For this review, take the finished solid that the model builds, in its own axes (mm). A direction names the side the tool comes from. Coordinates: 2 decimals unless noted, no trailing zeros. Order: outer loops, then holes, each group sorted by start corner. A loop starts at its lowest first (then second) coordinate and runs counter-clockwise, first axis right, second up. Notation, with made-up numbers: (81.25, 21) -> (140.25, 21) arc R33 ccw to (140.25, 60) -> close; hole circle Ø5 at (82, 22.5). An arc over 180 degrees is marked (long way). Write item = value, one per line. Start each with the question number.
1) Consider section A-A on y = 0. Give the boundary of the cut face in (x, z), and give its area (3 significant figures).
2) Machinability: for faces 1 (the face through (-4, 5, 2)), 2 (the face through (7, -4, 10)), 3 (the face through (4.93, -3.91, 7.46)), which of the approach directions +Z, -Z, +X, -X, +Y, -Y give a long, thin tool a straight path to every point of the face, cutting with its end or side? Answer none if there is none.
3) Insertion check: pin 1 Ø10 at (x, y) = (7.5, 6.5) entering from +Z; pin 2 Ø1.5 at (x, z) = (-5.5, 9) entering from +Y; pin 3 Ø5.5 at (y, z) = (3.5, 2.5) entering from -X; pin 4 Ø2.5 at (x, y) = (0, 0) entering from +Z. Each pin has a flat end and moves straight along its axis. Give the tip position at first contact, or say it passes through.
4) Wall thickness on probe 1 along Y at (x, z) = (0.25, 3.25); probe 2 along X at (y, z) = (9, 2.25); probe 3 along X at (y, z) = (3.75, 1.5): over which ranges is each line inside the solid? List them lowest first. Write a range as [from, to].
5) Consider section B-B on x = -9.25. Give the boundary of the cut face in (y, z), and give its area (3 significant figures).
6) Consider section C-C on x = 5.75. Give the boundary of the cut face in (y, z), and give its area (3 significant figures).
7) Draft analysis for pull direction X (two halves, no side actions). For faces 4 (the face through (0, 8, 10)), 5 (the face through (-11.99, 0.53, 2.54)), 6 (the face through (2.5, 0.2, 5)), state which applies: +X half, -X half, draft (parallel to the pull), parting line (faces both ways), or undercut.
8) Consider section D-D on z = 5.75. Give the boundary of the cut face in (x, y), and give its area (3 significant figures).
from build123d import *

# Parameters (mm, degrees)
BOSS_EXTRUDE1_DEPTH     = 5
SKETCH3_R               = 2
BOSS_EXTRUDE2_DEPTH     = 5
SKETCH4_R               = 2
CUT_EXTRUDE1_DEPTH      = 6
CUT_EXTRUDE1_DEPTH_BACK = 6
SKETCH5_R               = 12
SKETCH5_R_2             = 10
BOSS_EXTRUDE3_DEPTH     = 5


with BuildPart() as part:
    # Sketch1 → Boss-Extrude1 (new body)
    with BuildSketch(Plane.XY):
        with BuildLine():
            Line((4, 2.309401077), (4, 8))
            ThreePointArc((4, 8), (0, 12), (-4, 8))
            Line((-4, 8), (-4, 2.309401077))
            Line((-4, 2.309401077), (-8.92820323, -0.535898385))
            ThreePointArc((-8.92820323, -0.535898385), (-10.392304845, -6), (-4.92820323, -7.464101615))
            Line((-4.92820323, -7.464101615), (0, -4.618802154))
            Line((0, -4.618802154), (4.92820323, -7.464101615))
            ThreePointArc((4.92820323, -7.464101615), (10.392304845, -6), (8.92820323, -0.535898385))
            Line((8.92820323, -0.535898385), (4, 2.309401077))
        make_face()
    extrude(amount=BOSS_EXTRUDE1_DEPTH)

    # Sketch3 → Boss-Extrude2 (add)
    with BuildSketch(Plane.XY.offset(5)):
        with Locations((0, 8)):
            Circle(SKETCH3_R)
        with Locations((6.92820323, -4)):
            Circle(SKETCH3_R)
        with Locations((-6.92820323, -4)):
            Circle(SKETCH3_R)
        Circle(SKETCH3_R)
    extrude(amount=BOSS_EXTRUDE2_DEPTH)

    # Sketch4 → Cut-Extrude1 (cut, two sides)
    with BuildSketch(Plane.XY.offset(5)) as cut_extrude1_sk:
        Circle(SKETCH4_R)
    extrude(amount=CUT_EXTRUDE1_DEPTH, mode=Mode.SUBTRACT)
    extrude(cut_extrude1_sk.sketch, amount=-CUT_EXTRUDE1_DEPTH_BACK, mode=Mode.SUBTRACT)

    # Sketch5 → Boss-Extrude3 (add)
    with BuildSketch(Plane.XY.offset(5)):
        Circle(SKETCH5_R)
        Circle(SKETCH5_R_2, mode=Mode.SUBTRACT)
    extrude(amount=-BOSS_EXTRUDE3_DEPTH)


solid = part.part
Answer sheet:
q1.outline = (-12, 0) -> (-10, 0) -> (-10, 5) -> (-12, 5) -> close; (-8, 0) -> (-2, 0) -> (-2, 5) -> (-8, 5) -> close; (2, 0) -> (8, 0) -> (8, 5) -> (2, 5) -> close; (10, 0) -> (12, 0) -> (12, 5) -> (10, 5) -> close
q1.area = 80.0 mm2
q2.face_1 = +Z, -Z
q2.face_2 = +Z, +X, -X, +Y, -Y
q2.face_3 = +Z
q3.pin_1 = 5
q3.pin_2 = -2.12
q3.pin_3 = -11.98
q3.pin_4 = through
q4.probe_1 = [-12, -10], [-4.76, -1.98], [1.98, 12]
q4.probe_2 = [-7.94, -4.36], [-3.87, 3.87], [4.36, 7.94]
q4.probe_3 = [-11.4, -9.27], [-4, 4], [9.27, 11.4]
q5.outline = (-7.64, 0) -> (-0.74, 0) -> (-0.74, 5) -> (-7.64, 5) -> close; (3.8, 0) -> (7.64, 0) -> (7.64, 5) -> (3.8, 5) -> close
q5.area = 53.7 mm2
q6.outline = (-10.53, 0) -> (-8.18, 0) -> (-8.18, 5) -> (-10.53, 5) -> close; (-7.82, 0) -> (1.3, 0) -> (1.3, 5) -> (-2.38, 5) -> (-2.38, 10) -> (-5.62, 10) -> (-5.62, 5) -> (-7.82, 5) -> close; (8.18, 0) -> (10.53, 0) -> (10.53, 5) -> (8.18, 5) -> close
q6.area = 85.3 mm2
q7.face_4 = draft
q7.face_5 = parting line
q7.face_6 = undercut
q8.outline = circle Ø4 at (-6.93, -4); circle Ø4 at (0, 8); circle Ø4 at (6.93, -4)
q8.area = 37.7 mm2
